The model under review builds one solid part; all positions refer to its coordinate system, in mm. A direction names the side the tool comes from. Coordinates: 2 decimals unless noted, no trailing zeros. Order: outer loops, then holes, each group sorted by start corner. A loop starts at its lowest first (then second) coordinate and runs counter-clockwise, first axis right, second up. Notation, with made-up numbers: M -16,46 L 39,46 A29 cw 39,74 Z; hole C 47,-26 d3. An arc over 180 degrees is marked long. Answer as CSV lines item,"result". Start each with the question number.
Q1. Wall thickness on L1, parallel to Y at x = -15, z = 2 (3 decimals); L2, parallel to Y at x = 0, z = 3.8 (3 decimals); L3, parallel to Y at x = -0.5, z = 0.8: over which ranges is each line inside the solid? List them lowest first. Write a range as [from, to].
Q2. Consider section D-D on y = 21.5. Write out the cut boundary in (x, z), and give its area (3 significant figures).
Q3. The part is to be moulded in two halves that separate along X. For faces 6 (the face through (-23, 24, 3)), 7 (the face through (0, -25, 3)), 8 (the face through (-22, -3, 4)), say which applies: +X half, -X half, draft (parallel to the pull), parting line (faces both ways), or undercut.
Q4. Machinability: for faces 1 (the face through (-24, 0, 4)), 2 (the face through (17.307, -20.936, 4.891)), 3 (the face through (24, 23, 3)), 4 (the face through (-22.5, 0, 2)), 5 (the face through (0, -5, 6)), which of the approach directions +Z, -Z, +X, -X, +Y, -Y give a long, thin tool a straight path to every point of the face, cutting with its end or side? Answer none if there is none.
Q5. Consider section B-B on x = -15. Write out the cut boundary in (y, z) (3 decimals).
Q6. Consider section C-C on z = 1.5. State how many separate pieces and enclosed holes the cut face has, and give its area (3 significant figures).
Q7. Consider section A-A on y = -16.5. Write out the cut boundary in (x, z) (3 decimals).
Q8. For P1, Ø8, axis at x = 12, y = -7, coming from the -Z side; P2, Ø0.8, axis at x = 24, y = -1, coming from the +Z side; P3, Ø6, axis at x = -15, y = -16.5, coming from the +Z side, all flat-tipped, find the tip position at first contact; note any pin that passes through.
from build123d import *

# Parameters (mm, degrees)
F1_DEPTH  = 6
F2_W      = 2.5
F2_H      = 6
F3_DEPTH  = 2
F4_W      = 2.5
F4_H      = 6
F5_DEPTH  = 25
F6_R      = 2.375
F7_DEPTH  = 25
F8_R      = 2.375
F9_DEPTH  = 25
F10_R     = 6
F10_R_2   = 5
F11_DEPTH = 2.25
F12_R     = 3.95
F13_DEPTH = 25


with BuildPart() as f1:
    # F0 (on Top) → F1 (new body)
    with BuildSketch(Plane.XY):
        with BuildLine():
            ThreePointArc((-25, -20), (-23.535534, -23.535534), (-20, -25))
            Line((-20, -25), (20, -25))
            ThreePointArc((20, -25), (23.535534, -23.535534), (25, -20))
            Line((25, -20), (25, 20))
            ThreePointArc((25, 20), (23.535534, 23.535534), (20, 25))
            Line((20, 25), (-20, 25))
            ThreePointArc((-20, 25), (-23.535534, 23.535534), (-25, 20))
            Line((-25, 20), (-25, -20))
        make_face()
    extrude(amount=F1_DEPTH)

    # F2 (on face) → F3 (cut)
    with BuildSketch(Plane.XY.offset(6)):
        with Locations((-23.75, 0)):
            Rectangle(F2_W, F2_H)
        with Locations((23.75, 0)):
            Rectangle(F2_W, F2_H)
    extrude(amount=-F3_DEPTH, mode=Mode.SUBTRACT)

    # F4 (on face) → F5 (cut)
    with BuildSketch(Plane.XY.offset(6)):
        with Locations((-21.25, 0)):
            Rectangle(F4_W, F4_H)
        with Locations((21.25, 0)):
            Rectangle(F4_W, F4_H)
    extrude(amount=-F5_DEPTH, mode=Mode.SUBTRACT)

    # F6 (on face) → F7 (cut)
    with BuildSketch(Plane.XY.offset(6)):
        Circle(F6_R)
        with Locations((-10, 0)):
            Circle(F6_R)
        with Locations((0, -10)):
            Circle(F6_R)
        with Locations((10, 0)):
            Circle(F6_R)
        with Locations((0, 10)):
            Circle(F6_R)
    extrude(amount=-F7_DEPTH, mode=Mode.SUBTRACT)

    # F8 (on face) → F9 (cut)
    with BuildSketch(Plane.XY.offset(6)):
        with Locations((-15, -16.5)):
            Circle(F8_R)
        with Locations((15, -16.5)):
            Circle(F8_R)
        with Locations((-15, 16.5)):
            Circle(F8_R)
        with Locations((15, 16.5)):
            Circle(F8_R)
    extrude(amount=-F9_DEPTH, mode=Mode.SUBTRACT)

    # F10 (on face) → F11 (cut)
    with BuildSketch(Plane.XY.offset(6)):
        with Locations((-15, 16.5)):
            Circle(F10_R)
        with Locations((15, 16.5)):
            Circle(F10_R)
        with Locations((-15, -16.5)):
            Circle(F10_R_2)
        with Locations((15, -16.5)):
            Circle(F10_R_2)
    extrude(amount=-F11_DEPTH, mode=Mode.SUBTRACT)

    # F12 (on face) → F13 (cut)
    with BuildSketch(Plane.XY.offset(3.75)):
        with Locations((-15, 16.5)):
            Circle(F12_R)
        with Locations((15, 16.5)):
            Circle(F12_R)
    extrude(amount=-F13_DEPTH, mode=Mode.SUBTRACT)


solid = f1.part
Evaluation:
1,L1,"y = [-25, -18.875], [-14.125, 12.55], [20.45, 25]"
1,L2,"y = [-25, -12.375], [-7.625, -2.375], [2.375, 7.625], [12.375, 25]"
1,L3,"y = [-25, -12.32], [-7.68, -2.32], [2.32, 7.68], [12.32, 25]"
2,outline,"M -24.77,0 L 24.77,0 L 24.77,6 L 18.32,6 L 18.32,3.75 L 11.68,3.75 L 11.68,6 L -11.68,6 L -11.68,3.75 L -18.32,3.75 L -18.32,6 L -24.77,6 Z"
2,area,"267 mm²"
3,face 6,"-X half"
3,face 7,"draft"
3,face 8,"undercut"
4,face 1,"+Z, -X"
4,face 2,"+Z"
4,face 3,"+Z, -Z, +X, +Y"
4,face 4,"+Z, -Z"
4,face 5,"+Z, +X, -X, +Y, -Y"
5,outline,"M -25,0 L -18.875,0 L -18.875,3.75 L -21.5,3.75 L -21.5,6 L -25,6 Z; M -14.125,0 L 12.55,0 L 12.55,3.75 L 10.5,3.75 L 10.5,6 L -11.5,6 L -11.5,3.75 L -14.125,3.75 Z; M 20.45,0 L 25,0 L 25,6 L 22.5,6 L 22.5,3.75 L 20.45,3.75 Z"
6,separate pieces,"1"
6,enclosed holes,"11"
6,area,"2,230 mm²"
7,outline,"M -25,0 L -17.375,0 L -17.375,3.75 L -20,3.75 L -20,6 L -25,6 Z; M -12.625,0 L 12.625,0 L 12.625,3.75 L 10,3.75 L 10,6 L -10,6 L -10,3.75 L -12.625,3.75 Z; M 17.375,0 L 25,0 L 25,6 L 20,6 L 20,3.75 L 17.375,3.75 Z"
8,P1,"stops at z = 0"
8,P2,"stops at z = 4"
8,P3,"stops at z = 3.75"
